CAD build for the part. Positions are in the model's coordinates, mm. Face numbers are marked on the shaded views. A direction names the side the tool comes from. Coordinates: 2 decimals unless noted, no trailing zeros. Write each loop counter-clockwise with the first axis right and the second up, starting at its lowest first coordinate (ties: lowest second). Pieces come first, ordered by that corner, then holes. Notation, with made-up numbers: (25.25, 50.5) - (76.25, 50.5) arc R22 cw to (76.25, 86.5) - close; hole circle Ø6 at (-30.75, 3). An arc over 180 degrees is marked (long way). Answer in a Markdown table with one row per item. Add a question column.
Q1. Pin check, flat tips, straight feed: pin 1 (7.5 mm diameter, centred on x = 13, y = -7.5, fed in from +Z); pin 2 (1 mm diameter, centred on y = -9, z = 4, fed in from -X); pin 3 (9 mm diameter, centred on x = 44.5, z = 19.5, fed in from -Y); pin 4 (9 mm diameter, centred on x = 6.5, z = 22, fed in from +Y). Stop position of each tip, or through.
Q2. 3-axis set-ups, long thin cutter, end or side, ignore diameter. For the marked faces 1, 2, 3 and 4: which of +Z, -Z, +X, -X, +Y, -Y reach the whole face in a straight line?
Q3. Band-saw the part on A-A (z = 3). List the corners of the cut face in (x, y), and give its area (3 significant figures).
Q4. Band-saw the part on B-B (x = 20.5). List the corners of the cut face in (y, z).
Q5. Two-plate mould, pull along Y, no slides. Class the marked faces 5, 6, 7 and 8: +Y half, -Y half, draft (parallel to the pull), parting line (faces both ways), or undercut.
Q6. Band-saw the part on C-C (y = 12). List the corners of the cut face in (x, z).
Q7. Drill centre lines: line 1 along Z through (x, y) = (37, 15.5); line 2 along X through (y, z) = (8.5, 21.5); line 3 along Z through (x, y) = (13, 9.5). Where is each one in solid material? Low to high. Write a range as from..to.
Q8. Band-saw the part on D-D (z = 17). List the corners of the cut face in (x, y).
```python
from build123d import *

# Parameters (mm, degrees)
PAD_DEPTH       = 50
SKETCH001_W     = 35
SKETCH001_H     = 13
PAD001_DEPTH    = 25
POCKET_DEPTH    = 31.501
SKETCH003_W     = 5
SKETCH003_H     = 20
PAD002_DEPTH    = 18.5
POCKET001_DEPTH = 20.001
SKETCH005_W     = 5
SKETCH005_H     = 20
PAD003_DEPTH    = 18.5
POCKET002_DEPTH = 20.001


with BuildPart() as part:
    # Sketch → Pad (new body)
    with BuildSketch(Plane.YZ):
        Polygon((17.5, 0), (17.5, 13), (-17.5, 13), (-17.5, 0), (-10, 0), (-10, 8), (10, 8), (10, 0), align=None)
    extrude(amount=PAD_DEPTH)

    # Sketch001 (on Face2 of Pad) → Pad001 (join)
    with BuildSketch(Plane(origin=(0, 0, 13), x_dir=(0, -1, 0), z_dir=(0, 0, 1))):
        with Locations((0, 25)):
            Rectangle(SKETCH001_W, SKETCH001_H)
    extrude(amount=PAD001_DEPTH)

    # Sketch002 (on Face8 of Pad001) → Pocket (cut, through all)
    with BuildSketch(Plane.YZ.offset(31.5)):
        with BuildLine():
            Line((-17.5, 38), (-17.5, 18))
            Line((-17.5, 18), (-16.975592, 18))
            ThreePointArc((17.024408, 18), (0.024408, 34.999671), (-16.975592, 18))
            Line((17.5, 18), (17.024408, 18))
            Line((17.5, 18), (17.5, 38))
            Line((17.5, 38), (-17.5, 38))
        make_face()
    extrude(amount=-POCKET_DEPTH, mode=Mode.SUBTRACT)

    # Sketch003 (on Face2 of Pocket) → Pad002 (join)
    with BuildSketch(Plane.YZ.offset(31.5)):
        with Locations((0, 23)):
            Rectangle(SKETCH003_W, SKETCH003_H)
    extrude(amount=PAD002_DEPTH)

    # Sketch004 (on Face3 of Pad002) → Pocket001 (cut, through all)
    with BuildSketch(Plane(origin=(0, -2.5, 0), x_dir=(0, 0, -1), z_dir=(0, -1, 0))):
        Polygon((-33, 50), (-33, 31.5), (-13, 50), align=None)
    extrude(amount=-POCKET001_DEPTH, mode=Mode.SUBTRACT)

    # Sketch005 (on Face6 of Pocket001) → Pad003 (join)
    with BuildSketch(Plane(origin=(18.5, 0, 0), x_dir=(0, 1, 0), z_dir=(-1, 0, 0))):
        with Locations((0, -23)):
            Rectangle(SKETCH005_W, SKETCH005_H)
    extrude(amount=PAD003_DEPTH)

    # Sketch006 (on Face20 of Pad003) → Pocket002 (cut, through all)
    with BuildSketch(Plane(origin=(0, -2.5, 0), x_dir=(0, 0, -1), z_dir=(0, -1, 0))):
        Polygon((-33, 18.5), (-33, 0), (-13, 0), align=None)
    extrude(amount=-POCKET002_DEPTH, mode=Mode.SUBTRACT)


solid = part.part
```
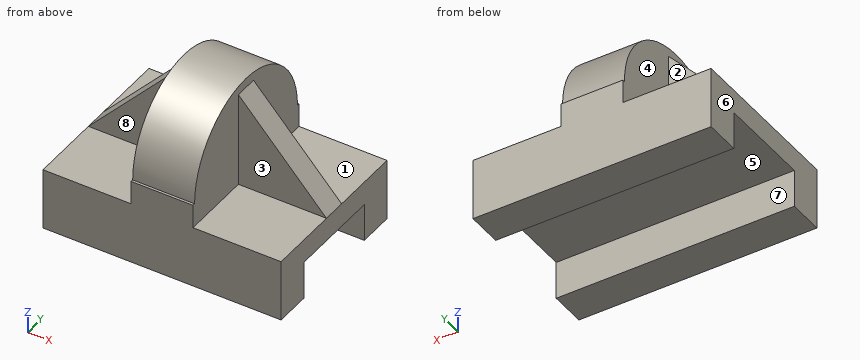
Checked values:
| question | item | result |
|---|---|---|
| 1 | pin 1 | stops at z = 13 |
| 1 | pin 2 | passes through |
| 1 | pin 3 | stops at y = -2.5 |
| 1 | pin 4 | stops at y = 2.5 |
| 2 | face 1 | +Z, +X, +Y |
| 2 | face 2 | +Z, -X, +Y |
| 2 | face 3 | +Z, +X, -Y |
| 2 | face 4 | +Z, -X |
| 3 | outline | (0, -17.5) - (50, -17.5) - (50, -10) - (0, -10) - close; (0, 10) - (50, 10) - (50, 17.5) - (0, 17.5) - close |
| 3 | area | 750 mm² |
| 4 | outline | (-17.5, 0) - (-10, 0) - (-10, 8) - (10, 8) - (10, 0) - (17.5, 0) - (17.5, 18) - (17.02, 18) arc R17 ccw to (-16.98, 18) - (-17.5, 18) - close |
| 5 | face 5 | undercut |
| 5 | face 6 | draft |
| 5 | face 7 | undercut |
| 5 | face 8 | -Y half |
| 6 | outline | (0, 0) - (50, 0) - (50, 13) - (31.5, 13) - (31.5, 30.07) - (18.5, 30.07) - (18.5, 13) - (0, 13) - close |
| 7 | line 1 | z = 0..13 |
| 7 | line 2 | x = 18.5..31.5 |
| 7 | line 3 | z = 8..13 |
| 8 | outline | (3.7, -2.5) - (18.5, -2.5) - (18.5, -17.5) - (31.5, -17.5) - (31.5, -2.5) - (46.3, -2.5) - (46.3, 2.5) - (31.5, 2.5) - (31.5, 17.5) - (18.5, 17.5) - (18.5, 2.5) - (3.7, 2.5) - close |
